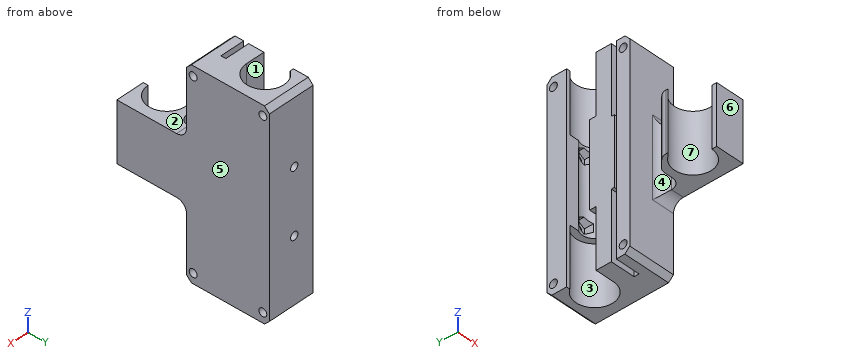
```python
from build123d import *

# Parameters (mm, degrees)
BOSS_EXTRUDE1_DEPTH      = 82
BOSS_EXTRUDE2_DEPTH      = 17
BOSS_EXTRUDE2_DEPTH_BACK = 17
CUT_EXTRUDE1_DEPTH       = 10
SKETCH6_R                = 1.6
CUT_EXTRUDE2_DEPTH       = 98.738426425
CUT_EXTRUDE3_DEPTH       = 14
CHAMFER1_SIZE            = 2
SKETCH9_W                = 29
SKETCH9_H                = 28.3
CUT_EXTRUDE4_DEPTH       = 98.738426425
FILLET1_R                = 4
FILLET2_R                = 4
CHAMFER2_SIZE            = 2
CHAMFER3_SIZE            = 5
FILLET3_R                = 4
CUT_EXTRUDE5_OUTLINE_W   = 1.6
CUT_EXTRUDE5_OUTLINE_H   = 7.954041593
CUT_EXTRUDE6_DEPTH       = 5


# Read off the part's stored shape, not the designer's step: Cut-Extrude5
with BuildPart() as part:
    # Sketch1 → Boss-Extrude1 (new body)
    with BuildSketch(Plane.XY):
        with BuildLine():
            Line((0, -47.6), (0, -49.6))
            Line((0, -49.6), (11.6, -49.6))
            Line((11.6, -49.6), (11.6, 12.4))
            Line((11.6, 12.4), (-7.6, 12.4))
            Line((-7.6, 12.4), (-7.6, 4.359180916))
            Line((-7.6, 4.359180916), (-6.225555537, 4.359180916))
            ThreePointArc((-6.225555537, 4.359180916), (6.741282332, 3.509289461), (0, -7.6))
            Line((0, -7.6), (-7.6, -7.6))
            Line((-7.6, -7.6), (-7.6, -9.6))
            Line((-7.6, -9.6), (-7.6, -18.625988463))
            Line((-7.6, -18.625988463), (-7.6, -36.851976926))
            Line((-7.6, -36.851976926), (-5.374011537, -34.625988463))
            ThreePointArc((-5.374011537, -34.625988463), (7.021484447, -37.091605914), (0, -47.6))
        make_face()
    extrude(amount=BOSS_EXTRUDE1_DEPTH)

    # Sketch2 → Boss-Extrude2 (add, two sides: drawn at the far end of the back side and taken through both)
    with BuildSketch(Plane(origin=(0, 0, 41), x_dir=(-1, 0, 0), z_dir=(0, 0, -1)).offset(-BOSS_EXTRUDE2_DEPTH_BACK)):
        with BuildLine():
            Line((0, -7.6), (7.6, -7.6))
            Line((7.6, -7.6), (7.6, -5))
            Line((7.6, -5), (0, -5))
            ThreePointArc((0, -5), (-4.837142988, 1.265720233), (2.448987901, 4.359180916))
            Line((2.448987901, 4.359180916), (6.225555537, 4.359180916))
            ThreePointArc((6.225555537, 4.359180916), (-6.741282332, 3.509289461), (0, -7.6))
        make_face()
    extrude(amount=BOSS_EXTRUDE2_DEPTH + BOSS_EXTRUDE2_DEPTH_BACK)

    # Sketch4 → Cut-Extrude1 (cut)
    with BuildSketch(Plane.ZY.offset(7.6)):
        Polygon((0, -13.8), (27.33, -13.8), (27.33, -15), (54.66, -15), (54.66, -13.8), (82, -13.8), (82, -15.8), (0, -15.8), align=None)
    extrude(amount=-CUT_EXTRUDE1_DEPTH, mode=Mode.SUBTRACT)

    # Sketch6 → Cut-Extrude2 (cut, through all)
    with BuildSketch(Plane.ZY.offset(7.6)):
        with Locations(Location((4, 9.74, 0), (0, 0, 270))):
            Circle(SKETCH6_R)
        with Locations(Location((4, -18.6, 0), (0, 0, 270))):
            Circle(SKETCH6_R)
    cut_extrude2 = extrude(amount=-CUT_EXTRUDE2_DEPTH, mode=Mode.SUBTRACT)

    # Mirror1: Cut-Extrude2 across plane
    add(cut_extrude2.mirror(Plane(origin=(0, 0, 41), x_dir=(1, 0, 0), z_dir=(0, 0, -1))), mode=Mode.SUBTRACT)

    # Sketch7 → Cut-Extrude3 (cut)
    with BuildSketch(Plane.ZY.offset(7.6)):
        Polygon((0, -29.4), (82, -29.4), (82, -21.3), (74, -21.3), (8, -21.3), (0, -21.3), align=None)
    extrude(amount=-CUT_EXTRUDE3_DEPTH, mode=Mode.SUBTRACT)

    # Chamfer1
    chamfer1_edges = [part.edges().sort_by_distance(p)[0] for p in [
        (2, 12.4, 0),
        (2, 12.4, 82),
    ]]
    chamfer(chamfer1_edges, length=CHAMFER1_SIZE)

    # Sketch9 → Cut-Extrude4 (cut, through all)
    with BuildSketch(Plane.ZY.offset(7.6)):
        with Locations((67.5, -35.45)):
            Rectangle(SKETCH9_W, SKETCH9_H)
        with Locations((14.5, -35.45)):
            Rectangle(SKETCH9_W, SKETCH9_H)
    extrude(amount=-CUT_EXTRUDE4_DEPTH, mode=Mode.SUBTRACT)

    # Fillet1
    fillet1_edges = [part.edges().sort_by_distance(p)[0] for p in [
        (6.4, -21.3, 41),
        (6.4, -29.4, 41),
    ]]
    fillet(fillet1_edges, radius=FILLET1_R)

    # Fillet2
    fillet2_edges = [part.edges().sort_by_distance(p)[0] for p in [
        (7, -21.3, 53),
        (7, -21.3, 29),
    ]]
    fillet(fillet2_edges, radius=FILLET2_R)

    # Chamfer2
    chamfer2_edges = [part.edges().sort_by_distance(p)[0] for p in [
        (2, -21.3, 0),
        (2, -21.3, 82),
    ]]
    chamfer(chamfer2_edges, length=CHAMFER2_SIZE)

    # Chamfer3
    chamfer3_edges = [part.edges().sort_by_distance(p)[0] for p in [
        (-7.6, -29.4, 41),
    ]]
    chamfer(chamfer3_edges, length=CHAMFER3_SIZE)

    # Fillet3
    fillet3_edges = [part.edges().sort_by_distance(p)[0] for p in [
        (-2.6, -29.4, 41),
        (-7.6, -34.4, 41),
    ]]
    fillet(fillet3_edges, radius=FILLET3_R)

    # Cut-Extrude5 outline → Cut-Extrude5 (revolve, cut)
    with BuildSketch(Plane(origin=(0.687222232, 0, 54), x_dir=(1, 0, 0), z_dir=(0, 0, 1))):
        with Locations((0.8, 8.422979204)):
            Rectangle(CUT_EXTRUDE5_OUTLINE_W, CUT_EXTRUDE5_OUTLINE_H)
    cut_extrude5 = revolve(axis=Axis((0.687222232, 0, 54), (0, 1, 0)), mode=Mode.SUBTRACT)

    # Mirror2: Cut-Extrude5 across plane
    add(cut_extrude5.mirror(Plane(origin=(0, 0, 41), x_dir=(1, 0, 0), z_dir=(0, 0, -1))), mode=Mode.SUBTRACT)

    # Sketch12 → Cut-Extrude6 (cut)
    with BuildSketch(Plane.XZ.offset(-2.396270795)):
        Polygon((-2.08405906, 52.4), (0.687222232, 50.8), (3.458503524, 52.4), (3.458503524, 55.6), (0.687222232, 57.2), (-2.08405906, 55.6), align=None)
    cut_extrude6 = extrude(amount=-CUT_EXTRUDE6_DEPTH, mode=Mode.SUBTRACT)

    # Mirror3: Cut-Extrude6 across plane
    add(cut_extrude6.mirror(Plane(origin=(0, 0, 41), x_dir=(1, 0, 0), z_dir=(0, 0, -1))), mode=Mode.SUBTRACT)


solid = part.part
```
Can you work these out from the model? Positions are in its coordinate system, mm. Face numbers are marked on the shaded views. A direction names the side the tool comes from. Round coordinates to 2 decimals unless told otherwise and drop trailing zeros. Loops run counter-clockwise (first coordinate to the right, second up) from the corner with the lowest first, then second, coordinate; pieces in that order, holes last. Notation, with made-up numbers: M 89,70.25 L 110,70.25 A20 ccw 110,88.25 Z; hole C -17.75,86.5 d3. An arc over 180 degrees is marked long. Answer in a Markdown table with one row per item.
1. Please list where these lines run through material, in increasing order: line 1 (Z direction, x = -3.5, y = -18.6); line 2 (Y direction, x = -0.75, z = 53.5); line 3 (Y direction, x = -3.5, z = 62.5). Write a range as from..to.
Established:
| item | result |
|---|---|
| line 1 | 0..2.4, 5.6..76.4, 79.6..82 |
| line 2 | -21.3..-15.8, -15..-5 |
| line 3 | -21.3..-15.8, -13.8..-7.6, 6.75..12.4 |
2. I'm going to push flat-ended pins straight in: pin 1 Ø5 at (x, z) = (-5, 11) entering from -Y; pin 2 Ø9.5 at (x, y) = (5, -32) entering from -Z; pin 3 Ø2 at (y, z) = (-49, 44.5) entering from -X; pin 4 Ø1.9 at (y, z) = (-18.6, 78) entering from -X. Where does each tip first touch, or does it pass through?
Established:
| item | result |
|---|---|
| pin 1 | y = -21.3 |
| pin 2 | z = 29 |
| pin 3 | x = 0 |
| pin 4 | through |
3. If we section it at B-B, the plane y = 0: Please give me the cut outline in (x, z), plus the area to 3 significant figures.
Established:
| item | result |
|---|---|
| outline | M 5,24 L 7.6,24 L 7.6,0 L 11.6,0 L 11.6,82 L 7.6,82 L 7.6,58 L 5,58 Z |
| area | 416 mm² |
4. On a 3-axis mill with a long thin cutter (end or side, diameter ignored), from which of +Z, -Z, +X, -X, +Y, -Y can I reach the whole of each face in a straight line? I mean the marked faces 1, 2, 3 and 4. Say none if no direction works.
Established:
| item | result |
|---|---|
| face 1 | +Z, -X |
| face 2 | +Z, +X, -X, -Y |
| face 3 | -Z |
| face 4 | +Z, -Z, -X |
5. If we section it at C-C, the plane x = 9.5: Please give me the cut outline in (y, z), plus the area to 3 significant figures.
Established:
| item | result |
|---|---|
| outline | M -49.6,29 L -25.3,29 A4 cw -21.3,25 L -21.3,2 L -19.3,0 L 10.4,0 L 12.4,2 L 12.4,80 L 10.4,82 L -19.3,82 L -21.3,80 L -21.3,57 A4 cw -25.3,53 L -49.6,53 Z; hole C -18.6,4 d3.2; hole C -18.6,78 d3.2; hole C 9.74,4 d3.2; hole C 9.74,78 d3.2 |
| area | 3,410 mm² |
6. Thinking about a two-plate mould opening in Y: for the marked faces 5, 6 and 7, which applies, pulls with the +Y half, pulls with the -Y half, needs draft (parallel to the pull), parting line crosses it, or undercut?
Established:
| item | result |
|---|---|
| face 5 | needs draft |
| face 6 | pulls with the -Y half |
| face 7 | undercut |
7. If we section it at A-A, the plane z = 4: Please give me the cut outline in (x, y).
Established:
| item | result |
|---|---|
| outline | M -7.6,-21.3 L 11.6,-21.3 L 11.6,-20.2 L -7.6,-20.2 Z; M -7.6,-17 L 11.6,-17 L 11.6,8.14 L -7.6,8.14 L -7.6,4.36 L -6.23,4.36 A7.6 cw long 0,-7.6 L -7.6,-7.6 L -7.6,-13.8 L 2.4,-13.8 L 2.4,-15.8 L -7.6,-15.8 Z; M -7.6,11.34 L 11.6,11.34 L 11.6,12.4 L -7.6,12.4 Z |
8. If we section it at D-D, the plane z = 73.5: Please give me the cut outline in (x, y), plus the area to 3 significant figures.
Established:
| item | result |
|---|---|
| outline | M -7.6,-21.3 L 11.6,-21.3 L 11.6,12.4 L -7.6,12.4 L -7.6,4.36 L -6.23,4.36 A7.6 cw long 0,-7.6 L -7.6,-7.6 L -7.6,-13.8 L 2.4,-13.8 L 2.4,-15.8 L -7.6,-15.8 Z |
| area | 431 mm² |
